Autodesk Inventor part; units mm, degrees
ref_plane "Work Plane1" through (12.7, 0, 0) normal (1, 0, 0) x (0, 0, -1)
ref_plane "YZ Plane" through (0, 0, 0) normal (1, 0, 0) x (0, 1, 0)
ref_plane "XZ Plane" through (0, 0, 0) normal (0, 1, 0) x (-1, 0, 0)
sketch "Sketch1" plane through (0, 0, 0) normal (0, 0, 1) x (1, 0, 0)
  line L0 (0, 0) -> (25.4, 0)
  line L1 (25.4, 0) -> (25.4, 82.55)
  line L2 (25.4, 82.55) -> (0, 82.55)
  line L3 (0, 82.55) -> (0, 0)
  line L4 (12.7, 82.55) -> (12.7, 0) construction
  circle A0 centre (12.7, 73.025) radius 1.5875
  circle A1 centre (12.7, 9.525) radius 1.5875
  dimension "d0" = 25.4
  dimension "d1" = 82.55
  dimension "d2" = 3.175
  dimension "d3" = 9.525
  dimension "d4" = 9.525
extrude "Extrusion1" add sketch "Sketch1" along normal blind 0.7937
ref_plane "Work Plane1" through (12.7, 0, 0) normal (1, 0, 0) x (0, 0, -1)
sketch "Sketch2" plane through (25.4, 0, 0) normal (1, 0, 0) x (0, 0, -1)
  line L0 (0, 0) -> (0, 82.55)
  line L1 (0, 82.55) -> (-0.7937, 82.55)
  line L2 (-0.7937, 0) -> (-0.7937, 82.55)
  line L3 (0, 0) -> (-0.7937, 0)
  line L4 (1.093, 107.9388) -> (-6.4365, 6.6182) construction
  line L5 (1.093, 107.9388) -> (127.7437, 98.527) construction
  line L6 (-0.7937, 82.55) -> (-2.2055, 63.5524)
  arc A0 (-2.2055, 63.5524) -> (-2.2278, 60.3774) centre (21.3863, 61.7992) ccw
  line L7 (-0.7937, 0) -> (-0.7937, 12.7)
  arc A1 (-0.7937, 12.7) -> (-2.2278, 60.3774) centre (-794.0664, 12.7) ccw
  line L8 (-0.7937, 82.55) -> (-0.0022, 82.4912)
  line L9 (-0.0022, 82.4912) -> (-1.4139, 63.4936)
  line L10 (-0.7937, 12.7) -> (0, 12.7) construction
  line L11 (-0.7937, 0) -> (0, 0)
  line L12 (0, 12.7) -> (0, 0)
  arc A2 (0, 12.7) -> (-1.4355, 60.4251) centre (-794.0664, 12.7) ccw
  arc A3 (-1.4139, 63.4936) -> (-1.4355, 60.4251) centre (21.3863, 61.7992) ccw
  dimension "d7" = 85.75
  dimension "d8" = 19.05
  dimension "d9" = 12.7
  dimension "d12" = 0.7937
  dimension "d15" = 101.6
  dimension "d16" = 127
  dimension "d17" = 25.4
  dimension "d30" = 3.175
extrude "Extrusion2" cut sketch "Sketch2" against normal blind 25.4 contours L3 L2 A2 L0 | A2 L2 L9 L8 L1 L0 | L8 L9 L2
extrude "Extrusion3" add sketch "Sketch2" against normal blind 25.4 contours L3 L2 A2 L0 | L2 A1 A0 L6 L9 A3 A2 | L8 L9 L2
sketch "Sketch3" plane through (25.4, 63.4936, 1.4139) normal (0, -0.0741085, -0.9972502) x (-1, 0, 0)
  line L0 (0, 0) -> (25.4, 0)
  line L1 (0, 19.05) -> (25.4, 19.05)
  line L2 (12.7, 19.05) -> (12.7, 0) construction
  circle A0 centre (12.7, 9.525) radius 1.5875
  point P0 (25.4, -63.2142)
  dimension "d22" = 3.175
  dimension "d23" = 9.525
extrude "Extrusion4" cut sketch "Sketch3" against normal through all
sketch "Sketch4" plane through (25.4, 0, 0) normal (0, 0, -1) x (-1, 0, 0)
  line L0 (0, 0) -> (25.4, 0)
  line L1 (0, 12.7) -> (25.4, 12.7)
  line L2 (12.7, 12.7) -> (12.7, 0) construction
  circle A0 centre (12.7, 9.525) radius 1.5875
  dimension "d26" = 3.175
  dimension "d27" = 9.525
extrude "Extrusion5" cut sketch "Sketch4" against normal through all
equation "\"d4\" = d3"
equation "\"d12\" = d11"
properties part number "Hopper to Pail Polycarbonate Flap Connector V2" material "Polycarbonate, Clear"
Work out the finished part from the listing and answer in its coordinate system (mm). A direction names the side the tool comes from. Give positions to 0.01 mm unless a question says otherwise; leave off trailing zeros. Loops run counter-clockwise (first coordinate to the right, second up) from the corner with the lowest first, then second, coordinate; pieces in that order, holes last. Notation, with made-up numbers: M 24,23 L 42,23 A26 ccw 42,42 Z; hole C 59.5,80 d2. An arc over 180 degrees is marked long. One line per item, written item: value. Start each with the question number.
1. Find the intervals of material crossed by probe 1 along Z at (x, y) = (10.75, 5); probe 2 along Z at (x, y) = (7.25, 26), in increasing order.
2. Each of these flat-tipped pins is pushed along its axis until it touches: P1, Ø4, axis at x = 3.5, y = 39.5, coming from the -Z side; P2, Ø1.5, axis at x = 22.5, y = 32.5, coming from the +Z side; P3, Ø6.5, axis at x = 11.5, y = 7, coming from the +Z side. Where does it stop, or does it pass through?
3. Find section D-D (y = 40). Give the vertices of the cut face in (x, z).
4. Which of the six approach directions +Z, -Z, +X, -X, +Y, -Y give full straight-line access (tool end or side, diameter ignored) to faces 4 (the face through (25.4, 41, 1)), 5 (the face through (12.88, 36.24, 0.35)), 6 (the face through (13, 6, 0.794))?
5. Determine the mould class of faces 1 (the face through (12.878, 75.295, 1.333)), 2 (the face through (12.88, 61.99, 2.27)), 3 (the face through (11.23, 72.42, 1.14)) for opening direction Y: released by +Y, released by -Y, zero draft, split by the parting line, or undercut.
6. Find section B-B (x = 12.7). Give the vertices of the cut face in (y, z).
7. Find section C-C (y = 28). Give the vertices of the cut face in (x, z), and give its area (3 significant figures).
8. Find section A-A (x = 22). Give the vertices of the cut face in (y, z).
Reported:
1. probe 1: z = 0 to 0.79
1. probe 2: z = 0.11 to 0.91
2. P1: stops at z = 0.39
2. P2: stops at z = 1.06
2. P3: stops at z = 0.79
3. outline: M 0,0.47 L 25.4,0.47 L 25.4,1.26 L 0,1.26 Z
4. face 4: +Z, -Z, +X, +Y, -Y
4. face 5: -Z, +X, -X
4. face 6: +Z, +X, -X, -Y
5. face 1: released by +Y
5. face 2: split by the parting line
5. face 3: undercut
6. outline: M 0,0 L 7.94,0 L 7.94,0.79 L 0,0.79 Z; M 11.11,0 L 12.7,0 A794.05 ccw 60.43,1.44 A22.88 cw 63.49,1.41 L 71.41,0.83 L 71.47,1.62 L 63.55,2.21 A23.66 ccw 60.38,2.23 A793.22 cw 12.7,0.79 L 11.11,0.79 Z; M 74.58,0.59 L 82.49,0 L 82.55,0.79 L 74.63,1.38 Z
7. outline: M 0,0.15 L 25.4,0.15 L 25.4,0.94 L 0,0.94 Z
7. area: 20.2 mm²
8. outline: M 0,0 L 12.7,0 A794.05 ccw 60.43,1.44 A22.88 cw 63.49,1.41 L 82.49,0 L 82.55,0.79 L 63.55,2.21 A23.66 ccw 60.38,2.23 A793.22 cw 12.7,0.79 L 0,0.79 Z
